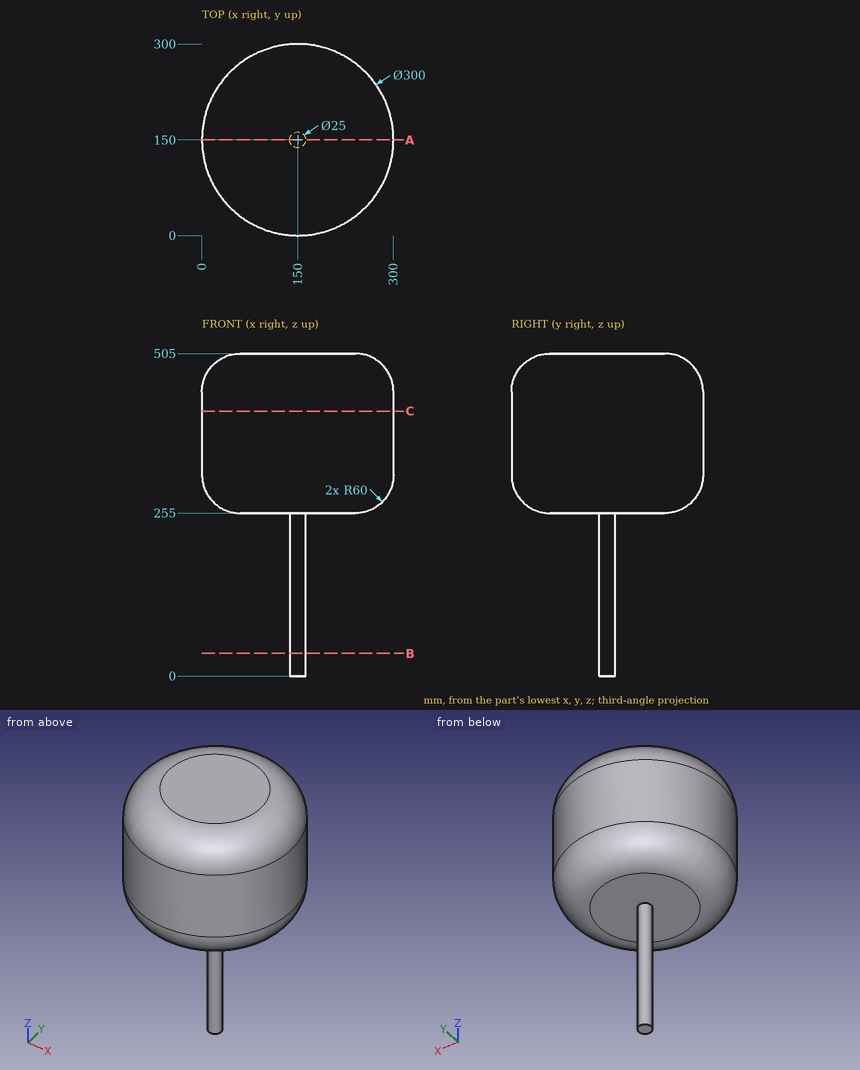
Verification items for this drawing (mm, ordinates from the low corner). Give positions to 0.01 mm unless a question says otherwise; leave off trailing zeros. Loops run counter-clockwise (first coordinate to the right, second up) from the corner with the lowest first, then second, coordinate; pieces in that order, holes last. Notation, with made-up numbers: M 79,-18.75 L 123,-18.75 A36 cw 123,16.25 Z; hole C -10,21 d3. An arc over 180 degrees is marked long. Answer as a JSON object with one key per item and string values. Group by question number.
Item 1: Material ranges on L1, parallel to Z at x = 126.5, y = 182; L2, parallel to X at y = 74, z = 404; L3, parallel to Y at x = 58.5, z = 337, recorded low to high.
Item 2: Sectioned sample at A-A on y = 150. Record the boundary of the cut face in (x, z), plus the area to 3 significant figures.
Item 3: Sectioned sample at C-C on z = 415. Record the boundary of the cut face in (x, y).
Item 4: Sectioned sample at B-B on z = 35.5. Record the boundary of the cut face in (x, y), plus the area to 3 significant figures.
Item 5: Gauge pin test, flat ends, axial feed: pin 1 (6 mm diameter, centred on x = 193.5, y = 48, fed in from -Z); pin 2 (4 mm diameter, centred on x = 107, y = 132.5, fed in from -Z); pin 3 (4 mm diameter, centred on x = 207, y = 246, fed in from -Z). Record the tip position at first contact, or that the pin passes through.
Findings below:
{
 "1": {"L1": "255 to 505", "L2": "20.68 to 279.32", "L3": "31.14 to 268.86"},
 "2": {"outline": "M 0,315 A60 ccw 60,255 L 137.5,255 L 137.5,0 L 162.5,0 L 162.5,255 L 240,255 A60 ccw 300,315 L 300,445 A60 ccw 240,505 L 60,505 A60 ccw 0,445 Z", "area": "78,300 mm2"},
 "3": {"outline": "C 150,150 d300"},
 "4": {"outline": "C 150,150 d25", "area": "491 mm2"},
 "5": {"pin 1": "z = 257.73", "pin 2": "z = 255", "pin 3": "z = 258.31"}
}
